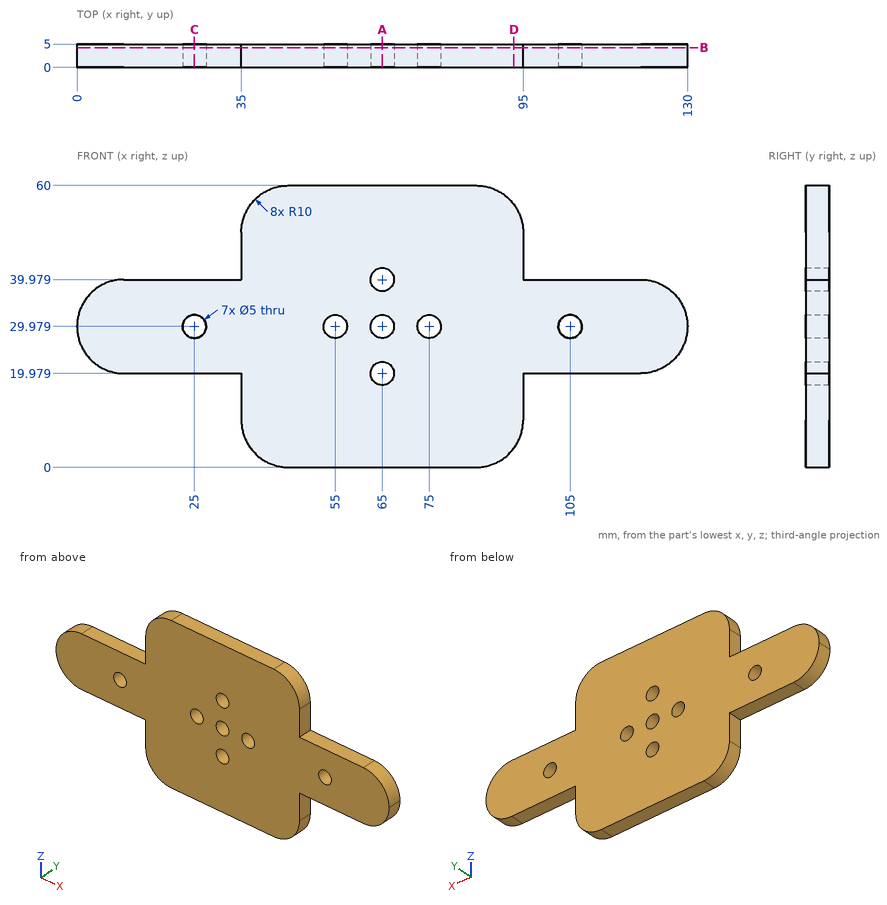
Answer from the drawing. Dimensions are ordinates in mm from the lowest x, y and z of the part. Give positions to 0.01 mm unless a question says otherwise; leave off trailing zeros. Order: outer loops, then holes, each group sorted by start corner. A loop starts at its lowest first (then second) coordinate and runs counter-clockwise, first axis right, second up. Notation, with made-up numbers: (3.5, 15.5) - (8.5, 15.5) arc R35 cw to (8.5, 51.5) - close; hole circle Ø1 at (-29.75, 50). An arc over 180 degrees is marked (long way). Use one line per item in the form item = value.
1) Each of these flat-tipped pins is pushed along its axis until it touches: pin 1 (1.5 mm diameter, centred on x = 19, y = 3.5, fed in from -Z); pin 2 (2.5 mm diameter, centred on x = 23, y = 1.5, fed in from +Z); pin 3 (1.5 mm diameter, centred on y = 2, z = 46.5, fed in from +X). Where does it stop, or does it pass through?
Verdict:
pin_1 = 19.98
pin_2 = 39.98
pin_3 = 95
2) Find section C-C on x = 25. Determine the outline of the cut face in (y, z), and give its area (3 significant figures).
Verdict:
outline = (0, 19.98) - (5, 19.98) - (5, 27.48) - (0, 27.48) - close; (0, 32.48) - (5, 32.48) - (5, 39.98) - (0, 39.98) - close
area = 75.0 mm^2
3) Consider probe 1 along Z at (x, y) = (65, 2.1); probe 2 along X at (y, z) = (2.45, 30); probe 3 along Z at (x, y) = (105, 1.8). Determine where each line is inside the solid, lowest interval first. Write a range as [from, to].
Verdict:
probe_1 = [0, 17.48], [22.48, 27.48], [32.48, 37.48], [42.48, 60]
probe_2 = [0, 22.5], [27.5, 52.5], [57.5, 62.5], [67.5, 72.5], [77.5, 102.5], [107.5, 130]
probe_3 = [19.98, 27.48], [32.48, 39.98]
4) Find section B-B on y = 4.25. Give the number of separate pieces and of enclosed holes in the cut face, and give its area (3 significant figures).
Verdict:
separate_pieces = 1
enclosed_holes = 7
area = 4,690 mm^2
5) Find section D-D on x = 93. Determine the outline of the cut face in (y, z), and give its area (3 significant figures).
Verdict:
outline = (0, 4) - (5, 4) - (5, 56) - (0, 56) - close
area = 260 mm^2
6) Find section A-A on x = 65. Determine the outline of the cut face in (y, z), and give its area (3 significant figures).
Verdict:
outline = (0, 0) - (5, 0) - (5, 17.48) - (0, 17.48) - close; (0, 22.48) - (5, 22.48) - (5, 27.48) - (0, 27.48) - close; (0, 32.48) - (5, 32.48) - (5, 37.48) - (0, 37.48) - close; (0, 42.48) - (5, 42.48) - (5, 60) - (0, 60) - close
area = 225 mm^2
